Build history of the part. All positions in model axes, mm. A direction names the side the tool comes from. Give positions to 0.01 mm unless a question says otherwise; leave off trailing zeros. Write each loop counter-clockwise with the first axis right and the second up, starting at its lowest first coordinate (ties: lowest second). Pieces come first, ordered by that corner, then holes.
from build123d import *

# Parameters (mm, degrees)
BOSS_EXTRUDE1_DEPTH = 19
CUT_EXTRUDE1_START  = -16
CUT_EXTRUDE1_DEPTH  = 32
MIRROR1_START       = -12.75
MIRROR1_DEPTH       = 5.5
MIRROR1_START_2     = 7.25
MIRROR1_2_DEPTH     = 5.5
MIRROR1_START_3     = -12.5
MIRROR1_3_DEPTH     = 5
MIRROR1_START_4     = 7.5
MIRROR1_4_DEPTH     = 5


# Read off the part's stored shape, not the designer's step: Mirror1
with BuildPart() as part:
    # Sketch1 → Boss-Extrude1 (new, symmetric)
    with BuildSketch(Plane.XY):
        Polygon((0, 0), (0, 36), (5.012193309, 36), (36, 5.012193309), (36, 0), align=None)
    extrude(amount=BOSS_EXTRUDE1_DEPTH, both=True)

    # Sketch2 → Cut-Extrude1 (cut)
    with BuildSketch(Plane.XY.offset(CUT_EXTRUDE1_START)):
        Polygon((5.5, 35.512193309), (5.5, 5.5), (35.512193309, 5.5), align=None)
    extrude(amount=CUT_EXTRUDE1_DEPTH, mode=Mode.SUBTRACT)

    # Mirror1 outline → Mirror1 (cut)
    with BuildSketch(Plane.XY.offset(MIRROR1_START)):
        Polygon((5.5, 12.472329862), (5.5, 29.5), (0, 29.5), (0, 6.363961031), align=None)
        Polygon((29.5, 5.5), (12.472329862, 5.5), (6.363961031, 0), (29.5, 0), align=None)
    extrude(amount=MIRROR1_DEPTH, mode=Mode.SUBTRACT)

    # Mirror1 2 outline → Mirror1 2 (cut)
    with BuildSketch(Plane.XY.offset(MIRROR1_START_2)):
        Polygon((5.5, 12.472329862), (5.5, 29.5), (0, 29.5), (0, 6.363961031), align=None)
        Polygon((29.5, 5.5), (12.472329862, 5.5), (6.363961031, 0), (29.5, 0), align=None)
    extrude(amount=MIRROR1_2_DEPTH, mode=Mode.SUBTRACT)

    # Mirror1 3 outline → Mirror1 3 (add)
    with BuildSketch(Plane.XY.offset(MIRROR1_START_3)):
        Polygon((35.3, 0), (32.999216572, 0), (32.072195597, -1.013438577), (33.043379246, -2), align=None)
        Polygon((-1.013438577, 32.072195597), (0, 32.999216572), (0, 35.3), (-2, 33.043379246), align=None)
        Polygon((0, 1.234750477), (0, 3.535533906), (-2, 1.278913151), (-1.013438577, 0.307729503), align=None)
        Polygon((1.278913151, -2), (3.535533906, 0), (1.234750477, 0), (0.307729503, -1.013438577), align=None)
    extrude(amount=MIRROR1_3_DEPTH)

    # Mirror1 4 outline → Mirror1 4 (add)
    with BuildSketch(Plane.XY.offset(MIRROR1_START_4)):
        Polygon((35.3, 0), (32.999216572, 0), (32.072195597, -1.013438577), (33.043379246, -2), align=None)
        Polygon((-1.013438577, 32.072195597), (0, 32.999216572), (0, 35.3), (-2, 33.043379246), align=None)
        Polygon((0, 1.234750477), (0, 3.535533906), (-2, 1.278913151), (-1.013438577, 0.307729503), align=None)
        Polygon((1.278913151, -2), (3.535533906, 0), (1.234750477, 0), (0.307729503, -1.013438577), align=None)
    extrude(amount=MIRROR1_4_DEPTH)


solid = part.part
(1) Probe line 1 (Z direction, x = 17.5, y = 2); line 2 (Z direction, x = 11.5, y = 20); line 3 (X direction, y = 31, z = -11.5). List the from-to ranges inside material, lowest first.
(2) Mould opens along Z. For faces 1 (the face through (-1, 2, 12.5)), 2 (the face through (29.5, 3, 10)), 3 (the face through (34.16, -1.01, 9.96)) say: +Z half, -Z half, draft (parallel to the pull), parting line (faces both ways), or undercut.
(3) Saw through at B-B, the plane x = 22. List the corners of the cut face in (y, z).
(4) 3-axis set-ups, long thin cutter, end or side, ignore diameter. For faces 4 (the face through (3, 29.5, 10)), 5 (the face through (-1, 33, 12.5)), 6 (the face through (-1, 2, -7.5)): which of +Z, -Z, +X, -X, +Y, -Y reach the whole face in a straight line?
(5) Saw through at D-D, the plane z = -2.5. List the corners of the cut face in (x, y), plus the area to 3 significant figures.
(6) Drop flat-ended pins along their axis: pin 1 (1 mm diameter, centred on x = -1.5, y = 1.5, fed in from +Z); pin 2 (8 mm diameter, centred on x = 14, z = -0.5, fed in from +Y); pin 3 (1 mm diameter, centred on x = 18, z = -5, fed in from -Y). Give the stop position or say it passes through.
(7) Saw through at A-A, the plane z = -9. Give the number of separate pieces and of enclosed holes in the cut face, plus the area to 3 significant figures.
(8) Saw through at C-C, the plane y = 18. List the corners of the cut face in (x, z), plus the area to 3 significant figures.
Computed values:
1. line 1: z = -19 to -12.75, -7.25 to 7.25, 12.75 to 19
1. line 2: z = -19 to -16, 16 to 19
1. line 3: x = 0 to 5.5
2. face 1: +Z half
2. face 2: undercut
2. face 3: draft
3. outline: (0, -19) - (19.01, -19) - (19.01, -16) - (5.5, -16) - (5.5, -12.75) - (0, -12.75) - close; (0, -7.25) - (5.5, -7.25) - (5.5, 7.25) - (0, 7.25) - close; (0, 12.75) - (5.5, 12.75) - (5.5, 16) - (19.01, 16) - (19.01, 19) - (0, 19) - close
4. face 4: +X, -X
4. face 5: +Z, -X, +Y, -Y
4. face 6: -X, +Y, -Y
5. outline: (0, 0) - (36, 0) - (36, 5.01) - (35.51, 5.5) - (5.5, 5.5) - (5.5, 35.51) - (5.01, 36) - (0, 36) - close
5. area: 366 mm2
6. pin 1: stops at z = 12.5
6. pin 2: stops at y = 5.5
6. pin 3: stops at y = 0
7. separate pieces: 3
7. enclosed holes: 0
7. area: 158 mm2
8. outline: (0, -19) - (23.01, -19) - (23.01, -16) - (5.5, -16) - (5.5, -12.75) - (0, -12.75) - close; (0, -7.25) - (5.5, -7.25) - (5.5, 7.25) - (0, 7.25) - close; (0, 12.75) - (5.5, 12.75) - (5.5, 16) - (23.01, 16) - (23.01, 19) - (0, 19) - close
8. area: 254 mm2
